Part model, mm, in its own coordinate system. Round coordinates to 2 decimals unless told otherwise and drop trailing zeros. Order: outer loops, then holes, each group sorted by start corner. A loop starts at its lowest first (then second) coordinate and runs counter-clockwise, first axis right, second up. Notation, with made-up numbers: (75, 88.25) - (87, 88.25) arc R12 cw to (87, 98.25) - close; hole circle Ø6 at (49.25, -15.5). An arc over 180 degrees is marked (long way). Answer as a JSON object with one key per item and string values.
```python
from build123d import *

# Parameters (mm, degrees)
F0_R     = 9.9
F1_DEPTH = 210
F2_SIZE  = 2
F3_R     = 2.5
F4_DEPTH = 8
F5_SIZE  = 0.5


with BuildPart() as f1:
    # F0 (on Top) → F1 (new body)
    with BuildSketch(Plane.XY):
        Circle(F0_R)
    extrude(amount=F1_DEPTH)

    # F2
    f2_edges = [f1.edges().sort_by_distance(p)[0] for p in [
        (-9.9, 0, 210),
    ]]
    chamfer(f2_edges, length=F2_SIZE)

    # F3 (on face) → F4 (cut)
    with BuildSketch(Plane(origin=(0, 0, 0), x_dir=(1, 0, 0), z_dir=(0, 0, -1))):
        Circle(F3_R)
    extrude(amount=-F4_DEPTH, mode=Mode.SUBTRACT)

    # F5
    f5_edges = [f1.edges().sort_by_distance(p)[0] for p in [
        (-9.9, 0, 0),
    ]]
    chamfer(f5_edges, length=F5_SIZE)


solid = f1.part
```
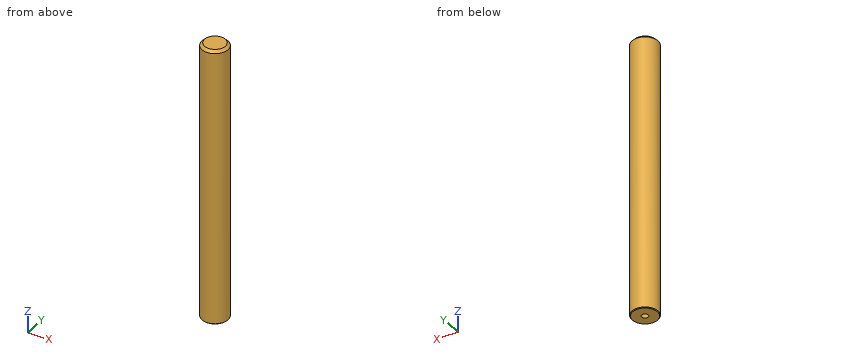
Item 1: Cut at A-A (z = 43.5). Write the cut outline in (x, y).
Taken from the geometry:
{"outline": "circle Ø19.8 at (0, 0)"}
Item 2: Probe L1, parallel to Y at x = 0, z = 2.75; L2, parallel to Y at x = 0, z = 79. List the from-to ranges inside material, lowest first. Write a range as from..to.
Taken from the geometry:
{"L1": "-9.9..-2.5, 2.5..9.9", "L2": "-9.9..9.9"}
Item 3: Drop flat-ended pins along their axis: P1, Ø3, axis at x = -7, z = 170.5, coming from the +Y side; P2, Ø3, axis at x = 0, y = 0, coming from the -Z side; P3, Ø6, axis at x = 6.5, z = 62.5, coming from the -Y side. Give the stop position or say it passes through.
Taken from the geometry:
{"P1": "y = 8.23", "P2": "z = 8", "P3": "y = -9.26"}
